Verification items for the finished model (mm, model axes). A direction names the side the tool comes from. Round coordinates to 2 decimals unless told otherwise and drop trailing zeros. Order: outer loops, then holes, each group sorted by start corner. A loop starts at its lowest first (then second) coordinate and runs counter-clockwise, first axis right, second up. Notation, with made-up numbers: (30.5, 60) -> (83.5, 60) arc R35 ccw to (83.5, 96) -> close; hole circle Ø9 at (-1.5, -0.5). An arc over 180 degrees is marked (long way). Return JSON: item names as keys, results as strings. Group by question number.
Item 1: Scan lines: probe 1 along X at (y, z) = (5, -7); probe 2 along X at (y, z) = (22, -10); probe 3 along Y at (x, z) = (19.5, 0). Record each from-to range of solid material in increasing order. Write a range as from..to.
Item 2: Sectioned sample at D-D on x = -19. Record the cut outline in (y, z).
Item 3: Draft check along Y on faces 6 (the flat face through (0, 58.5, -11)), 7 (the cylindrical face through (22.482, 57.871, -11.57)), 8 (the flat face through (-14, 36, -6.5)), 9 (the flat face through (0, 0, 0)). Enter one of: pulls with the +Y half, pulls with the -Y half, needs draft (parallel to the pull), parting line crosses it, or undercut.
Item 4: Sectioned sample at A-A on x = 0. Record the cut outline in (y, z).
Item 5: Sectioned sample at C-C on y = 22. Record the cut outline in (x, z).
Item 6: Access from +Z, -Z, +X, -X, +Y, -Y to the whole of each face (thin tool, end or side, straight path). Record for faces 1 (the flat face through (25, 17, 0)), 2 (the flat face through (0, 38, -15)), 3 (the flat face through (-12, 8, -7)), 4 (the cylindrical face through (-6.2, 5.1, 0)), 5 (the cylindrical face through (-1.409, 41.855, -15.74)).
Item 7: Depth check by flat-ended pin: pin 1 Ø5 at (x, y) = (21, 50.5) entering from +Z; pin 2 Ø1.7 at (x, z) = (-12, -7.5) entering from -Y; pin 3 Ø10 at (x, z) = (-13, 9) entering from +Y. Enter the tip coordinate at first touch or a pass-through.
Item 8: Sectioned sample at B-B on z = 13.5. Record the cut outline in (x, y).
```python
from build123d import *

# Parameters (mm, degrees)
SKETCH2_W           = 60
SKETCH2_H           = 33
BOSS_EXTRUDE1_DEPTH = 65
SKETCH3_W           = 23
SKETCH3_H           = 57
CUT_EXTRUDE1_DEPTH  = 60
SKETCH4_W           = 21
SKETCH4_H           = 41
CUT_EXTRUDE2_DEPTH  = 8.5
SKETCH4_3_R         = 1.3
CUT_EXTRUDE3_DEPTH  = 11
SKETCH6_R           = 3
SKETCH6_R_2         = 1
CUT_EXTRUDE4_DEPTH  = 66
FILLET2_R           = 25
FILLET4_R           = 25
BOSS_EXTRUDE2_DEPTH = 5
SKETCH9_R           = 6.5
CUT_EXTRUDE5_DEPTH  = 2.5
SKETCH10_R          = 10.5
CUT_EXTRUDE6_DEPTH  = 2.3
SKETCH12_R          = 1
CUT_EXTRUDE7_DEPTH  = 5.7


with BuildPart() as part:
    # Sketch2 → Boss-Extrude1 (new body)
    with BuildSketch(Plane(origin=(0, 0, 0), x_dir=(1, 0, 0), z_dir=(0, 1, 0))):
        Rectangle(SKETCH2_W, SKETCH2_H)
    extrude(amount=BOSS_EXTRUDE1_DEPTH)

    # Sketch3 → Cut-Extrude1 (cut)
    with BuildSketch(Plane.ZY.offset(30)):
        with Locations((5, 36.5)):
            Rectangle(SKETCH3_W, SKETCH3_H)
    extrude(amount=-CUT_EXTRUDE1_DEPTH, mode=Mode.SUBTRACT)

    # Sketch4 → Cut-Extrude2 (cut)
    with BuildSketch(Plane.XY.offset(-6.5)):
        with Locations((0, 38)):
            Rectangle(SKETCH4_W, SKETCH4_H)
    extrude(amount=-CUT_EXTRUDE2_DEPTH, mode=Mode.SUBTRACT)

    # Sketch4<3> → Cut-Extrude3 (cut, through all)
    with BuildSketch(Plane.XY.offset(-6.5)):
        with Locations((5, 14)):
            Circle(SKETCH4_3_R)
        with Locations((-5, 62)):
            Circle(SKETCH4_3_R)
        with Locations((5, 62)):
            Circle(SKETCH4_3_R)
        with Locations((-5, 14)):
            Circle(SKETCH4_3_R)
    extrude(amount=-CUT_EXTRUDE3_DEPTH, mode=Mode.SUBTRACT)

    # Sketch6 → Cut-Extrude4 (cut, through all)
    with BuildSketch(Plane.XZ):
        with Locations((-12.2, 0)):
            Circle(SKETCH6_R)
        with Locations((-19.2, 0)):
            Circle(SKETCH6_R_2)
        with Locations((-5.2, 0)):
            Circle(SKETCH6_R_2)
        with Locations((-12.2, 7)):
            Circle(SKETCH6_R_2)
    extrude(amount=-CUT_EXTRUDE4_DEPTH, mode=Mode.SUBTRACT)

    # Fillet2
    fillet2_edges = [part.edges().sort_by_distance(p)[0] for p in [
        (-30, 65, -11.5),
    ]]
    fillet(fillet2_edges, radius=FILLET2_R)

    # Fillet4
    fillet4_edges = [part.edges().sort_by_distance(p)[0] for p in [
        (30, 65, -11.5),
    ]]
    fillet(fillet4_edges, radius=FILLET4_R)

    # Sketch8 → Boss-Extrude2 (add)
    with BuildSketch(Plane.ZY.offset(30)):
        Polygon((-6.5, 40), (16.5, 8), (-6.5, 8), align=None)
    boss_extrude2 = extrude(amount=-BOSS_EXTRUDE2_DEPTH)

    # Mirror1: Boss-Extrude2 across plane
    add(boss_extrude2.mirror(Plane(origin=(0, 0, 0), x_dir=(0, 0, 1), z_dir=(1, 0, 0))))

    # Sketch9 → Cut-Extrude5 (cut, through all)
    with BuildSketch(Plane.XY.offset(-15)):
        with Locations((0, 48.2)):
            Circle(SKETCH9_R)
    extrude(amount=-CUT_EXTRUDE5_DEPTH, mode=Mode.SUBTRACT)

    # Sketch10 → Cut-Extrude6 (cut)
    with BuildSketch(Plane.XZ):
        with Locations((-12.2, 0)):
            Circle(SKETCH10_R)
    extrude(amount=-CUT_EXTRUDE6_DEPTH, mode=Mode.SUBTRACT)

    # Sketch12 → Cut-Extrude7 (cut)
    with BuildSketch(Plane.XZ.offset(-2.3)):
        with Locations((-12.35085129, -7)):
            Circle(SKETCH12_R)
    extrude(amount=-CUT_EXTRUDE7_DEPTH, mode=Mode.SUBTRACT)


solid = part.part
```
Recorded:
{
 "1": {"probe 1": "-30..-13.35, -11.35..30", "probe 2": "-30..-10.5, 10.5..30", "probe 3": "0..8"},
 "2": {"outline": "(0, -16.5) -> (60.71, -16.5) -> (60.71, -6.5) -> (8, -6.5) -> (8, -0.98) -> (2.3, -0.98) -> (2.3, -8) -> (0, -8) -> close; (0, 8) -> (2.3, 8) -> (2.3, 0.98) -> (8, 0.98) -> (8, 16.5) -> (0, 16.5) -> close"},
 "3": {"face 6": "undercut", "face 7": "pulls with the +Y half", "face 8": "needs draft", "face 9": "pulls with the -Y half"},
 "4": {"outline": "(0, -16.5) -> (41.7, -16.5) -> (41.7, -15) -> (17.5, -15) -> (17.5, -6.5) -> (8, -6.5) -> (8, 16.5) -> (0, 16.5) -> close; (54.7, -16.5) -> (65, -16.5) -> (65, -6.5) -> (58.5, -6.5) -> (58.5, -15) -> (54.7, -15) -> close"},
 "5": {"outline": "(-30, -16.5) -> (30, -16.5) -> (30, 6.44) -> (25, 6.44) -> (25, -6.5) -> (10.5, -6.5) -> (10.5, -15) -> (-10.5, -15) -> (-10.5, -6.5) -> (-25, -6.5) -> (-25, 6.44) -> (-30, 6.44) -> close"},
 "6": {"face 1": "+Z, +Y", "face 2": "+Z", "face 3": "-Y", "face 4": "+Y, -Y", "face 5": "+Z, -Z"},
 "7": {"pin 1": "z = -6.5", "pin 2": "y = 2.3", "pin 3": "y = 8"},
 "8": {"outline": "(-30, 0) -> (30, 0) -> (30, 12.17) -> (25, 12.17) -> (25, 8) -> (-25, 8) -> (-25, 12.17) -> (-30, 12.17) -> close"}
}
